Verification items for this drawing (mm, ordinates from the low corner). A direction names the side the tool comes from. Give positions to 0.01 mm unless a question says otherwise; leave off trailing zeros. Order: outer loops, then holes, each group sorted by start corner. A loop starts at its lowest first (then second) coordinate and runs counter-clockwise, first axis right, second up.
(1) Gauge pin test, flat ends, axial feed: pin 1 (4 mm diameter, centred on y = 66, z = 85, fed in from -X); pin 2 (1 mm diameter, centred on x = 149, y = 11, fed in from -Z); pin 3 (15 mm diameter, centred on x = 180.29, z = 23.5, fed in from -Y); pin 4 (3.5 mm diameter, centred on y = 42, z = 110.5, fed in from -X) (1 decimal). Record the tip position at first contact, or that the pin passes through.
(2) Sectioned sample at A-A on z = 70. Record the cut outline in (x, y), plus the area to 3 significant figures.
(3) Scan lines: L1, parallel to X at y = 6, z = 23 (1 decimal); L2, parallel to Y at x = 46.5, z = 104; L3, parallel to Z at x = 101.5, y = 25.5 (1 decimal). Record each from-to range of solid material in increasing order.
(4) Mould release check, pull along Z, two halves, no side actions. Record for the marked faces 1, 2 and 3: pulls with the +Z half, pulls with the -Z half, needs draft (parallel to the pull), parting line crosses it, or undercut.
(5) Sectioned sample at D-D on z = 23.5. Record the cut outline in (x, y) (1 decimal).
(6) Access from +Z, -Z, +X, -X, +Y, -Y to the whole of each face (thin tool, end or side, straight path). Record for the marked faces 4, 5 and 6.
(7) Sectioned sample at B-B on y = 8.5. Count the separate pieces of the cut face and the enclosed holes in it, plus the area to 3 significant figures.
(8) Sectioned sample at C-C on y = 46.5. Record the cut outline in (x, z).
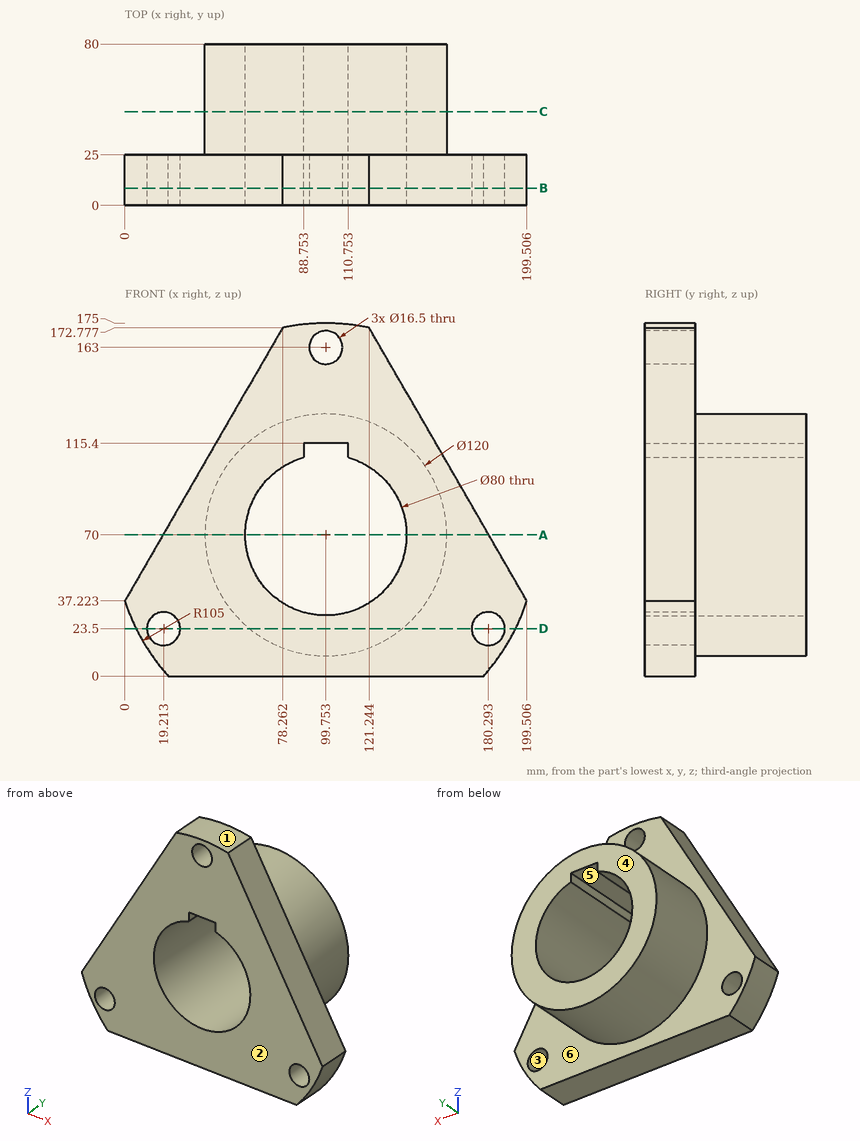
Ans:
1. pin 1: stops at x = 41.18
1. pin 2: stops at z = 0
1. pin 3: passes through
1. pin 4: stops at x = 53.9
2. outline: (18.92, 0) - (59.75, 0) - (59.75, 80) - (39.75, 80) - (39.75, 25) - (18.92, 25) - close; (139.75, 0) - (180.58, 0) - (180.58, 25) - (159.75, 25) - (159.75, 80) - (139.75, 80) - close
2. area: 4,240 mm2
3. L1: x = 5.9 to 11, 27.4 to 172.1, 188.5 to 193.6
3. L2: y = 0 to 25
3. L3: z = 10 to 30, 115.4 to 130
4. face 1: pulls with the +Z half
4. face 2: needs draft
4. face 3: undercut
5. outline: (5.6, 0) - (11, 0) - (11, 25) - (5.6, 25) - close; (27.5, 0) - (172, 0) - (172, 25) - (137.7, 25) - (137.7, 80) - (61.8, 80) - (61.8, 25) - (27.5, 25) - close; (188.5, 0) - (193.9, 0) - (193.9, 25) - (188.5, 25) - close
6. face 4: +Z, -Z, +X, -X, +Y
6. face 5: +Y, -Y
6. face 6: +Y
7. separate pieces: 1
7. enclosed holes: 4
7. area: 17,500 mm2
8. outline: circle Ø120 at (99.75, 70); hole (88.75, 108.46) arc R40 ccw (long way) to (110.75, 108.46) - (110.75, 115.4) - (88.75, 115.4) - close
